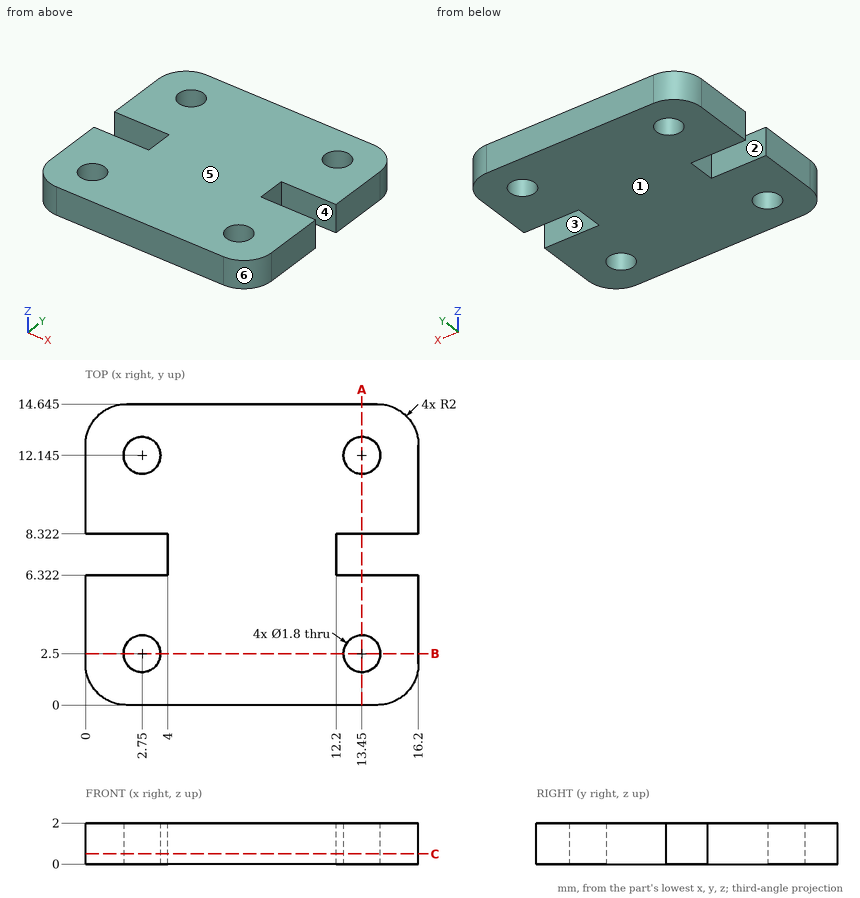
Here's the drawing with two shaded views (mm, measured from the low corner). I have some questions. A direction names the side the tool comes from. Give positions to 0.01 mm unless a question says otherwise; leave off trailing zeros. Write each loop counter-clockwise with the first axis right and the second up, starting at its lowest first coordinate (ties: lowest second). Pieces come first, ordered by that corner, then holes. Notation, with made-up numbers: (61, -0.5) - (83, -0.5) arc R15 cw to (83, 26.5) - close; hole circle Ø10 at (45.5, 26.25). An arc over 180 degrees is marked (long way). One line per item, written item: value. Start each with the question number.
Item 1: Imagine slicing it at B-B, the plane y = 2.5. List the corners of the cut face in (x, z) for me.
Item 2: If we mould it in two halves opening along Y, with no side actions, what happens to the marked faces 4, 5 and 6? For each: +Y half, -Y half, draft (parallel to the pull), parting line (faces both ways), or undercut.
Item 3: Imagine slicing it at C-C, the plane z = 0.5. Give the number of separate pieces and of enclosed holes in the cut face, and give its area (3 significant figures).
Item 4: Imagine slicing it at A-A, the plane x = 13.45. List the corners of the cut face in (y, z) for me (1 decimal), and give its area (3 significant figures).
Item 5: Which directions (+Z, -Z, +X, -X, +Y, -Y) give clear straight access to the entire face, cutting with the end or side of a thin tool? Please do the marked faces 1, 2 and 3.
Item 6: Please list where these lines run through material, in increasing order: line 1 (Y direction, x = 2.75, z = 0.75) (1 decimal); line 2 (X direction, y = 2.5, z = 1.45); line 3 (Y direction, x = 14.5, z = 1.55). Write a range as from..to.
Item 7: I'm going to push flat-ended pins straight in: pin 1 (1.6 mm diameter, centred on x = 2.75, y = 12.145, fed in from -Z); pin 2 (1 mm diameter, centred on y = 7.5, z = 1.5, fed in from -X). Where does each tip first touch, or does it pass through?
Geometry says:
1. outline: (0, 0) - (1.85, 0) - (1.85, 2) - (0, 2) - close; (3.65, 0) - (12.55, 0) - (12.55, 2) - (3.65, 2) - close; (14.35, 0) - (16.2, 0) - (16.2, 2) - (14.35, 2) - close
2. face 4: undercut
2. face 5: draft
2. face 6: -Y half
3. separate pieces: 1
3. enclosed holes: 4
3. area: 208 mm^2
4. outline: (0, 0) - (1.6, 0) - (1.6, 2) - (0, 2) - close; (3.4, 0) - (6.3, 0) - (6.3, 2) - (3.4, 2) - close; (8.3, 0) - (11.2, 0) - (11.2, 2) - (8.3, 2) - close; (13, 0) - (14.6, 0) - (14.6, 2) - (13, 2) - close
4. area: 18.1 mm^2
5. face 1: -Z, +X, -X, +Y, -Y
5. face 2: +Z, -Z, -X
5. face 3: +Z, -Z, +X
6. line 1: 0..1.6, 3.4..6.3, 8.3..11.2, 13..14.6
6. line 2: 0..1.85, 3.65..12.55, 14.35..16.2
6. line 3: 0.02..6.32, 8.32..14.62
7. pin 1: through
7. pin 2: x = 4
